Source: three-view drawing plus pictorial views. Frame: mm from the lowest corner of the part. A direction names the side the tool comes from. Coordinates: 2 decimals unless noted, no trailing zeros. Loops run counter-clockwise (first coordinate to the right, second up) from the corner with the lowest first, then second, coordinate; pieces in that order, holes last. Notation, with made-up numbers: M -35.5,-31.75 L -2.5,-31.75 A24 ccw -2.5,-13.75 Z; hole C 73,-30.5 d5. An arc over 180 degrees is marked long. Use a Markdown table: item, result. Add a question column.
1. Draft query along Z for the marked faces 3, 4 and 5. Return one class per face: +Z half, -Z half, draft (parallel to the pull), parting line (faces both ways), or undercut.
2. Pin query (flat end, axial travel): pin 1 (1.5 mm diameter, centred on y = 29.5, z = 4, fed in from +X); pin 2 (1 mm diameter, centred on y = 28.5, z = 2.5, fed in from -X); pin 3 (4 mm diameter, centred on x = 4, y = 32.5, fed in from +Z). Return the tip coordinate at first contact, or that it passes through.
3. Section B-B on z = 3. Output: boundary loops of the cut face in (x, y), then the cut area to 4 significant figures.
4. Section A-A on x = 3.5. Output: boundary loops of the cut face in (y, z).
5. Section C-C on y = 13. Output: boundary loops of the cut face in (x, z), then the cut area to 3 significant figures.
6. Line query: L1, parallel to Y at x = 5.5, z = 1.25; L2, parallel to Z at x = 2.5, y = 6.5. Output: solid intervals per line, ascending. Write a range as [from, to].
7. Set-up query: the marked faces 1 and 2. Return all of +Z, -Z, +X, -X, +Y, -Y with unobstructed straight access to the full face (end or side cutting, diameter ignored); none if empty.
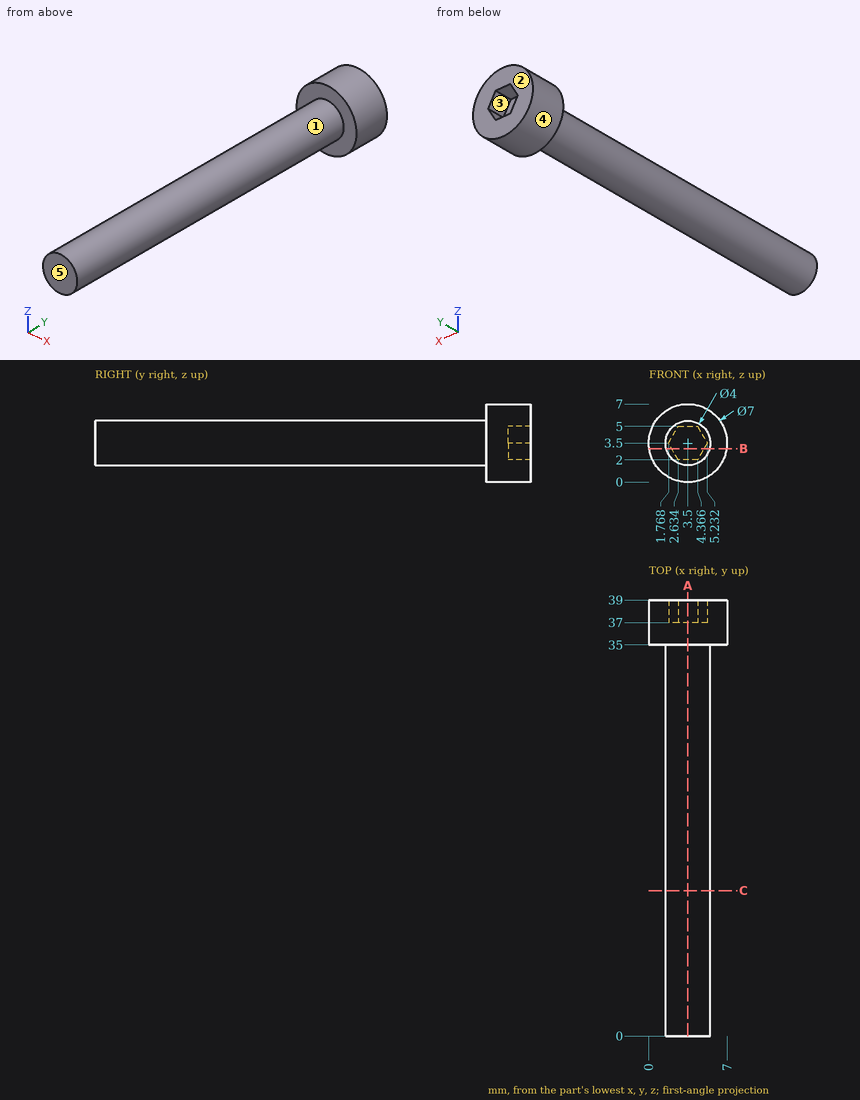
Answers below:
| question | item | result |
|---|---|---|
| 1 | face 3 | undercut |
| 1 | face 4 | parting line |
| 1 | face 5 | draft |
| 2 | pin 1 | stops at x = 5.5 |
| 2 | pin 2 | stops at x = 1.56 |
| 2 | pin 3 | stops at z = 5.5 |
| 3 | outline | M 0.04,35 L 1.56,35 L 1.56,0 L 5.44,0 L 5.44,35 L 6.96,35 L 6.96,39 L 4.94,39 L 4.94,37 L 2.06,37 L 2.06,39 L 0.04,39 Z |
| 3 | area | 157.5 mm² |
| 4 | outline | M 0,1.5 L 35,1.5 L 35,0 L 39,0 L 39,2 L 37,2 L 37,5 L 39,5 L 39,7 L 35,7 L 35,5.5 L 0,5.5 Z |
| 5 | outline | C 3.5,3.5 d4 |
| 5 | area | 12.6 mm² |
| 6 | L1 | y = [35, 39] |
| 6 | L2 | z = [1.77, 5.23] |
| 7 | face 1 | -Y |
| 7 | face 2 | +Z, -Z, +X, -X, +Y |
